```python
from build123d import *

# Parameters (mm, degrees)
PROFILEBOSS_EXTRUDE1_DEPTH    = 4.3
ANGLESKETCH7_W                = 10.25
ANGLESKETCH7_H                = 2
ANGLEBOSS_EXTRUDE3_DEPTH      = 5.5
UNDERROLLERSKETCH10_W         = 6.25
UNDERROLLERSKETCH10_H         = 2
UNDERROLLERCUT_EXTRUDE5_DEPTH = 16.714565224
UNDERFILLET22_R               = 1
OPENNINGCUT_EXTRUDE1_REACH    = 17.715
SKETCH2_W                     = 2.0625
SKETCH2_H                     = 2
OUTCHAMFER1_SIZE              = 2
TOPFILLET1_R                  = 1
CLAMPMOUNTHOLESKETCH3_R       = 2.05
CUT_EXTRUDE1_DEPTH            = 4.1


with BuildPart() as part:
    # Sketch1 → ProfileBoss-Extrude1 (new body)
    with BuildSketch(Plane(origin=(0, 0, 0), x_dir=(1, 0, 0), z_dir=(0, 1, 0))):
        with BuildLine():
            Line((10.25, 4), (10.25, 0))
            Line((10.25, 0), (0, 0))
            Line((0, 0), (0, 4))
            ThreePointArc((0, 4), (5.125, 6.770898034), (10.25, 4))
        make_face()
    extrude(amount=PROFILEBOSS_EXTRUDE1_DEPTH)

    # AngleSketch7 → AngleBoss-Extrude3 (add)
    with BuildSketch(Plane(origin=(0, 4.3, 0), x_dir=(1, 0, 0), z_dir=(0, 1, 0))):
        with Locations((5.125, 1)):
            Rectangle(ANGLESKETCH7_W, ANGLESKETCH7_H)
    extrude(amount=ANGLEBOSS_EXTRUDE3_DEPTH)

    # UnderRollerSketch10 → UnderRollerCut-Extrude5 (cut, through all)
    with BuildSketch(Plane.XY):
        with Locations((5.125, 7.3)):
            Rectangle(UNDERROLLERSKETCH10_W, UNDERROLLERSKETCH10_H)
    extrude(amount=-UNDERROLLERCUT_EXTRUDE5_DEPTH, mode=Mode.SUBTRACT)

    # UnderFillet22
    underfillet22_edges = [part.edges().sort_by_distance(p)[0] for p in [
        (5.125, 8.3, -2),
    ]]
    fillet(underfillet22_edges, radius=UNDERFILLET22_R)

    # Sketch2 → OpenningCut-Extrude1 (cut, up to next)
    with BuildSketch(Plane(origin=(0, 9.8, 0), x_dir=(1, 0, 0), z_dir=(0, 1, 0)), mode=Mode.PRIVATE) as openningcut_extrude1_sk1:
        with Locations((5.125, 1)):
            Rectangle(SKETCH2_W, SKETCH2_H)
    openningcut_extrude1_tool1 = extrude(openningcut_extrude1_sk1.sketch, amount=-OPENNINGCUT_EXTRUDE1_REACH, mode=Mode.PRIVATE) & part.part
    add(openningcut_extrude1_tool1.solids().sort_by_distance((5.125, 9.8, -1))[0], mode=Mode.SUBTRACT)

    # OutChamfer1
    outchamfer1_edges = [part.edges().sort_by_distance(p)[0] for p in [
        (5.125, 6.3, 0),
    ]]
    chamfer(outchamfer1_edges, length=OUTCHAMFER1_SIZE - 0.0001)  # a hair under: the kernel refuses the full size

    # TopFillet1
    topfillet1_edges = [part.edges().sort_by_distance(p)[0] for p in [
        (8.203125, 9.8, -2),
        (2.046875, 9.8, -2),
    ]]
    fillet(topfillet1_edges, radius=TOPFILLET1_R)

    # ClampMountHoleSketch3 → Cut-Extrude1 (cut)
    with BuildSketch(Plane.XZ):
        with Locations(Location((5.125, -4, 0), (0, 0, 270))):
            Circle(CLAMPMOUNTHOLESKETCH3_R)
    extrude(amount=-CUT_EXTRUDE1_DEPTH, mode=Mode.SUBTRACT)


solid = part.part
```
The model under review builds one solid part; all positions refer to its coordinate system, in mm. A direction names the side the tool comes from. Coordinates: 2 decimals unless noted, no trailing zeros. Write each loop counter-clockwise with the first axis right and the second up, starting at its lowest first coordinate (ties: lowest second). Pieces come first, ordered by that corner, then holes. Notation, with made-up numbers: (86, 89) -> (95, 89) arc R23 ccw to (95, 113) -> close; hole circle Ø7 at (53, 26.5). An arc over 180 degrees is marked (long way). One line per item, written item: value. Start each with the question number.
Q1. Add section D-D, the plane z = -0.75. Give the boundary of the cut face in (x, y).
Q2. The part is to be moulded in two halves that separate along X. For faces 1 (the face through (0, 4, -2)), 2 (the face through (3, 8.3, -0.5)), 3 (the face through (5, 4.3, -4)), 4 (the face through (10.25, 4, -2)), say which applies: +X half, -X half, draft (parallel to the pull), parting line (faces both ways), or undercut.
Q3. To check wall thickness, follow probe 1 along Z at (x, y) = (1, 8.5); probe 2 along Y at (x, z) = (6, -4.5); probe 3 along Y at (x, z) = (7, -5.75). State the ranges of each line that lie inside material, in increasing order.
Q4. Add section A-A, the plane y = 7. Give the boundary of the cut face in (x, z), then the cut area to 3 significant figures.
Q5. Add section C-C, the plane y = 2.25. Give the boundary of the cut face in (x, z) (3 decimals), then the cut area to 3 significant figures.
Q6. Clearance check with flat-ended pins moving along their axes: P1, Ø1.6, axis at y = 9, z = -0.5, coming from the -X side; P2, Ø3.5, axis at x = 5.125, z = -4, coming from the +Y side; P3, Ø3.5, axis at x = 2.5, y = 7.5, coming from the -Z side; P4, Ø1.2, axis at x = 4.5, z = -4, coming from the -Y side. State where each tip first meets the part, or that it passes through.
Q7. For faces 5 (the face through (5, 4.1, -4)), 6 (the face through (7.2, 8.5, -1.6)), 7 (the face through (7.2, 8.3, -0.5)), list the 3-axis set-ups (+Z, -Z, +X, -X, +Y, -Y) from which the entire face can be reached by the end or side of a thin tool; tool diameter is ignored.
Response:
1. outline: (0, 0) -> (10.25, 0) -> (10.25, 9.8) -> (6.16, 9.8) -> (6.16, 8.3) -> (8.25, 8.3) -> (8.25, 5.05) -> (2, 5.05) -> (2, 8.3) -> (4.09, 8.3) -> (4.09, 9.8) -> (0, 9.8) -> close
2. face 1: -X half
2. face 2: undercut
2. face 3: draft
2. face 4: +X half
3. probe 1: -2 to 0
3. probe 2: 4.1 to 4.3
3. probe 3: 0 to 4.3
4. outline: (0, -2) -> (2, -2) -> (2, 0) -> (0, 0) -> close; (8.25, -2) -> (10.25, -2) -> (10.25, 0) -> (8.25, 0) -> close
4. area: 8.00 mm²
5. outline: (0, -4) arc R6.125 ccw to (10.25, -4) -> (10.25, 0) -> (0, 0) -> close; hole circle Ø4.1 at (5.125, -4)
5. area: 47.8 mm²
6. P1: x = 0
6. P2: y = 4.3
6. P3: z = -2
6. P4: y = 4.1
7. face 5: -Y
7. face 6: -Z
7. face 7: +Z, -Z
